CAD build for the part. Positions are in the model's coordinates, mm. A direction names the side the tool comes from. Coordinates: 2 decimals unless noted, no trailing zeros. Order: outer loops, then holes, each group sorted by start corner. A loop starts at its lowest first (then second) coordinate and runs counter-clockwise, first axis right, second up.
from build123d import *

# Parameters (mm, degrees)
F0_W     = 5
F0_H     = 3
F1_DEPTH = 2.5


with BuildPart() as f1:
    # F0 (on Top) → F1 (new body, symmetric)
    with BuildSketch(Plane.XY):
        Polygon((135, 26.49), (-135, 26.49), (-135, 23.49), (-135, -26.49), (135, -26.49), (135, 23.49), align=None)
        with Locations((137.5, 24.99)):
            Rectangle(F0_W, F0_H)
        with Locations((-137.5, 24.99)):
            Rectangle(F0_W, F0_H)
    extrude(amount=F1_DEPTH, both=True)


solid = f1.part
1) Drill centre line: probe 1 along X at (y, z) = (-11.5, -1.45). Where is it in solid material? Low to high.
2) Which spindle directions (+Z, -Z, +X, -X, +Y, -Y) get a long thin tool onto all of the face, cutting with end or side? Do faces 1 (the flat face through (-2, 0, 2.5)), 2 (the flat face through (135, -2, 0)), 3 (the flat face through (-135, -1, 0)). Say none if no direction does.
3) Pin check, flat tips, straight feed: P1, Ø1.5, axis at x = -137.5, z = 0, coming from the -Y side; P2, Ø3, axis at y = -9.5, z = -2, coming from the +X side; P3, Ø3, axis at y = -0.5, z = -1.5, coming from the -X side. Stop position of each tip, or through.
4) Slice it at B-B (y = -15). List the corners of the cut face in (x, z), plus the area to 3 significant figures.
5) Slice it at A-A (z = 0.15). List the corners of the cut face in (x, y).
Worked out:
1. probe 1: x = -135 to 135
2. face 1: +Z, +X, -X, +Y, -Y
2. face 2: +Z, -Z, +X, -Y
2. face 3: +Z, -Z, -X, -Y
3. P1: stops at y = 23.49
3. P2: stops at x = 135
3. P3: stops at x = -135
4. outline: (-135, -2.5) - (135, -2.5) - (135, 2.5) - (-135, 2.5) - close
4. area: 1,350 mm2
5. outline: (-140, 23.49) - (-135, 23.49) - (-135, -26.49) - (135, -26.49) - (135, 23.49) - (140, 23.49) - (140, 26.49) - (-140, 26.49) - close
